Autodesk Inventor part; units mm, degrees
ref_plane "YZ Plane" through (0, 0, 0) normal (1, 0, 0) x (0, 1, 0)
ref_plane "XZ Plane" through (0, 0, 0) normal (0, 1, 0) x (-1, 0, 0)
ref_plane "XY Plane" through (0, 0, 0) normal (0, 0, 1) x (1, 0, 0)
sketch "Sketch1" plane through (0, 0, 0) normal (0, 0, 1) x (1, 0, 0)
  line L0 (0, -50) -> (-18, -50)
  line L1 (-18, -50) -> (-18, 50)
  line L2 (-18, 50) -> (18, 50)
  line L3 (18, 50) -> (18, -50)
  line L4 (18, -50) -> (0, -50)
  circle A0 centre (0, 0) radius 9
extrude "Extrusion2" add sketch "Sketch1" along normal blind 8
sketch "Sketch3" plane through (0, 0, 8) normal (0, 0, 1) x (1, 0, 0)
  line L0 (-18, 0) -> (18, 0) construction
  line L1 (18, 50) -> (18, -50) construction
  line L2 (-18, 50) -> (-18, -50) construction
  line L3 (-18, -50) -> (18, -50)
  line L4 (-18, -50) -> (18, -50)
  line L5 (18, -50) -> (18, -38)
  line L6 (18, -38) -> (-18, -38)
  line L7 (-18, -38) -> (-18, -50)
  line L8 (18, 50) -> (-18, 50)
  line L9 (-18, 50) -> (18, 50)
  line L10 (18, 50) -> (18, 38)
  line L11 (18, 38) -> (-18, 38)
  line L12 (-18, 38) -> (-18, 50)
  point P0 (0, 0)
  point P1 (-11, -27)
  point P2 (11.0001, -26.9664)
  point P3 (-11, 27)
  point P4 (11.0001, 26.9664)
  dimension "d57" = 36
  dimension "d58" = 12
  dimension "d59" = 36
  dimension "d60" = 12
hole "Hole1" at (-11, -27, 8) at (11.0001, -26.9664, 8) at (-11, 27, 8) at (11.0001, 26.9664, 8) direction (0, 0, -1) diameter 3.4 end through all
sketch "Sketch6" plane through (0, 0, 0) normal (0, 0, -1) x (-1, 0, 0)
  circle A0 centre (-11, -11) radius 2.9
  circle A1 centre (11, -11) radius 2.9
  circle A2 centre (11, 11) radius 2.9
  circle A3 centre (-11, 11) radius 2.9
  point P0 (0, 0)
extrude "Extrusion5" cut sketch "Sketch6" against normal through all
sketch "Sketch7" plane through (0, 0, 0) normal (0, 0, -1) x (-1, 0, 0)
  circle A0 centre (-11, -11) radius 2.9
  circle A1 centre (-11, -11) radius 5
  circle A2 centre (-11, 11) radius 2.9
  circle A3 centre (-11, 11) radius 5
  circle A4 centre (11, 11) radius 2.9
  circle A5 centre (11, 11) radius 5
  circle A6 centre (11, -11) radius 2.9
  circle A7 centre (11, -11) radius 5
  point P0 (0, 0)
  dimension "d44" = 10
  dimension "d45" = 10
  dimension "d46" = 10
  dimension "d47" = 10
extrude "Extrusion6" cut sketch "Sketch7" against normal blind 5
sketch "Sketch8" plane through (0, 0, 8) normal (0, 0, 1) x (1, 0, 0)
  line L0 (-18, 50) -> (-18, -50)
  line L1 (18, -49.142) -> (18, -37.142)
  line L2 (18, -37.142) -> (-18, -37.142)
  line L3 (-18, -37.142) -> (-18, -49.142)
  line L4 (18, 49.142) -> (18, 37.142)
  line L5 (18, 37.142) -> (-18, 37.142)
  line L6 (-18, 37.142) -> (-18, 49.142)
  line L7 (-18, -50) -> (18, -50)
  line L8 (18, -37.142) -> (-18, -37.142)
  line L9 (-18, -37.142) -> (-18, -50)
  line L10 (-18, -50) -> (18, -50)
  line L11 (18, -50) -> (18, -37.142)
  line L12 (-18, 50) -> (18, 50)
  line L13 (18, 37.142) -> (-18, 37.142)
  line L14 (-18, 37.142) -> (-18, 50)
  line L15 (-18, 50) -> (18, 50)
  line L16 (18, 50) -> (18, 37.142)
  point P0 (0, 0)
  dimension "d61" = 36
  dimension "d62" = 12
  dimension "d63" = 36
  dimension "d64" = 12
extrude "Extrusion7" cut sketch "Sketch8" against normal through all
properties part number "MOJ KOLNIERZ" material "Stainless Steel, Austenitic"
The listing builds one solid part. Answer for the finished solid, in the listing's coordinates (mm). A direction names the side the tool comes from. Give positions to 0.01 mm unless a question says otherwise; leave off trailing zeros. Order: outer loops, then holes, each group sorted by start corner. A loop starts at its lowest first (then second) coordinate and runs counter-clockwise, first axis right, second up. Notation, with made-up numbers: (-19.5, -7.75) - (26.5, -7.75) arc R11 cw to (26.5, 11.25) - close; hole circle Ø10 at (60, -23). An arc over 180 degrees is marked (long way). One line per item, written item: value. Start each with the question number.
1) Given pin 1 Ø3.5 at (x, y) = (-11, -11) entering from -Z (3 decimals); pin 2 Ø9.5 at (x, y) = (11, -11) entering from -Z, each flat-ended and moving along its own axis, determine where each tip first touches the part or whether it passes through.
2) The mould has two halves that part along Y. Classify faces 3 (the face through (0, 37.142, 4)), 4 (the face through (-4, 9, 0)), 5 (the face through (12.035, -25.617, 3.944)): released by +Y, released by -Y, zero draft, split by the parting line, or undercut.
3) Find the intervals of material crossed by L1, parallel to Y at x = 11, z = 1.1; L2, parallel to Y at x = 11, z = 6.9; L3, parallel to Y at x = 7, z = 1.25, in increasing order.
4) A cutting plane is placed at D-D on x = 1.5. Give the vertices of the cut face in (y, z), then the cut area to 3 significant figures.
5) A cutting plane is placed at C-C on y = -11. Give the vertices of the cut face in (x, z), then the cut area to 3 significant figures.
6) A tool of negligible diameter and unlimited length cuts with its end or side. For faces 1 (the face through (-13.2, 8.8, 5)), 2 (the face through (-10.35, 25.43, 3.94)), from which of +Z, -Z, +X, -X, +Y, -Y can it reach the whole face along a straight path? Write none if from no direction.
7) A cutting plane is placed at A-A on y = 0. Give the vertices of the cut face in (x, z).
8) A cutting plane is placed at B-B on x = -11. Give the vertices of the cut face in (y, z).
Answer sheet:
1. pin 1: passes through
1. pin 2: stops at z = 5
2. face 3: released by +Y
2. face 4: zero draft
2. face 5: undercut
3. L1: y = -37.14 to -28.67, -25.27 to -16, -6 to 6, 16 to 25.27, 28.67 to 37.14
3. L2: y = -37.14 to -28.67, -25.27 to -13.9, -8.1 to 8.1, 13.9 to 25.27, 28.67 to 37.14
3. L3: y = -37.14 to -14, -8 to -5.66, 5.66 to 8, 14 to 37.14
4. outline: (-37.14, 0) - (-8.87, 0) - (-8.87, 8) - (-37.14, 8) - close; (8.87, 0) - (37.14, 0) - (37.14, 8) - (8.87, 8) - close
4. area: 452 mm2
5. outline: (-18, 0) - (-16, 0) - (-16, 5) - (-13.9, 5) - (-13.9, 8) - (-18, 8) - close; (-8.1, 5) - (-6, 5) - (-6, 0) - (6, 0) - (6, 5) - (8.1, 5) - (8.1, 8) - (-8.1, 8) - close; (13.9, 5) - (16, 5) - (16, 0) - (18, 0) - (18, 8) - (13.9, 8) - close
5. area: 153 mm2
6. face 1: -Z
6. face 2: +Z, -Z
7. outline: (-18, 0) - (-9, 0) - (-9, 8) - (-18, 8) - close; (9, 0) - (18, 0) - (18, 8) - (9, 8) - close
8. outline: (-37.14, 0) - (-28.7, 0) - (-28.7, 8) - (-37.14, 8) - close; (-25.3, 0) - (-16, 0) - (-16, 5) - (-13.9, 5) - (-13.9, 8) - (-25.3, 8) - close; (-8.1, 5) - (-6, 5) - (-6, 0) - (6, 0) - (6, 5) - (8.1, 5) - (8.1, 8) - (-8.1, 8) - close; (13.9, 5) - (16, 5) - (16, 0) - (25.3, 0) - (25.3, 8) - (13.9, 8) - close; (28.7, 0) - (37.14, 0) - (37.14, 8) - (28.7, 8) - close
